from build123d import *

# Parameters (mm, degrees)
CROQUIS1_R              = 0.5
SALIENTE_EXTRUIR2_DEPTH = 0.2


with BuildPart() as part:
    # Croquis1 → Saliente-Extruir2 (new body)
    with BuildSketch(Plane.XY):
        with BuildLine():
            Line((-1.620168748, 6), (-0.633616905, 0.401284958))
            ThreePointArc((-0.633616905, 0.401284958), (0, -0.75), (0.633616905, 0.401284958))
            Line((0.633616905, 0.401284958), (1.620168748, 6))
            Line((1.620168748, 6), (0, 10))
            Line((0, 10), (-1.620168748, 6))
        make_face()
        Circle(CROQUIS1_R, mode=Mode.SUBTRACT)
    extrude(amount=SALIENTE_EXTRUIR2_DEPTH)


solid = part.part
Here's how the part is built. I have some questions about the finished solid (model axes, mm). Coordinates: 2 decimals unless noted, no trailing zeros. Write each loop counter-clockwise with the first axis right and the second up, starting at its lowest first coordinate (ties: lowest second). Pieces come first, ordered by that corner, then holes.
Item 1: I want a section at A-A on y = 0. Write out the boundary of the cut face in (x, z).
Item 2: I want a section at D-D on x = -1.35. Write out the boundary of the cut face in (y, z).
Item 3: If I drill on line 1 (X direction, y = 4.5, z = 0.15); line 2 (X direction, y = 2.5, z = 0.15), over which ranges is the centre line in solid material (lowest first)?
Item 4: I want a section at B-B on z = 0.05. Write out the boundary of the cut face in (x, y).
Item 5: I want a section at C-C on x = -0.4. Write out the boundary of the cut face in (y, z), and give its area (3 significant figures).
Findings below:
1. outline: (-0.75, 0) - (-0.5, 0) - (-0.5, 0.2) - (-0.75, 0.2) - close; (0.5, 0) - (0.75, 0) - (0.75, 0.2) - (0.5, 0.2) - close
2. outline: (4.47, 0) - (6.67, 0) - (6.67, 0.2) - (4.47, 0.2) - close
3. line 1: x = -1.36 to 1.36
3. line 2: x = -1 to 1
4. outline: (-1.62, 6) - (-0.63, 0.4) arc R0.75 ccw (long way) to (0.63, 0.4) - (1.62, 6) - (0, 10) - close; hole circle Ø1 at (0, 0)
5. outline: (-0.63, 0) - (-0.3, 0) - (-0.3, 0.2) - (-0.63, 0.2) - close; (0.3, 0) - (9.01, 0) - (9.01, 0.2) - (0.3, 0.2) - close
5. area: 1.81 mm2
